```python
from build123d import *

# Parameters (mm, degrees)
SKETCH1_W                  = 25.4
SKETCH1_H                  = 25.4
BOSS_EXTRUDE1_DEPTH        = 6.35
SKETCH2_R                  = 3.175
CUT_EXTRUDE1_DEPTH         = 20.05
F_6_32_TAPPED_HOLE1_REACH  = 31.099
F_6_32_TAPPED_HOLE1_BORE_R = 1.35255


with BuildPart() as part:
    # Sketch1 → Boss-Extrude1 (new body)
    with BuildSketch(Plane(origin=(0, 0, 0), x_dir=(1, 0, 0), z_dir=(0, 1, 0))):
        Rectangle(SKETCH1_W, SKETCH1_H)
    extrude(amount=BOSS_EXTRUDE1_DEPTH)

    # Sketch2 → Cut-Extrude1 (cut, through all)
    with BuildSketch(Plane(origin=(0, 6.35, 0), x_dir=(1, 0, 0), z_dir=(0, 1, 0))):
        with Locations(Location((0, 0, 0), (0, 0, 270))):
            Circle(SKETCH2_R)
    extrude(amount=-CUT_EXTRUDE1_DEPTH, mode=Mode.SUBTRACT)

    # #6-32 Tapped Hole1 bore → #6-32 Tapped Hole1 (cut, up to next)
    with BuildSketch(Plane(origin=(0, 0, -12.7), x_dir=(-1, 0, 0), z_dir=(0, 0, -1)), mode=Mode.PRIVATE) as f_6_32_tapped_hole1_sk1:
        with Locations((0, 3.175)):
            Circle(F_6_32_TAPPED_HOLE1_BORE_R)
    f_6_32_tapped_hole1_tool1 = extrude(f_6_32_tapped_hole1_sk1.sketch, amount=-F_6_32_TAPPED_HOLE1_REACH, mode=Mode.PRIVATE) & part.part
    add(f_6_32_tapped_hole1_tool1.solids().sort_by_distance((0, 3.175, -12.7))[0], mode=Mode.SUBTRACT)


solid = part.part
```
Design review of the part built by this model. Coordinates are the model's own, in mm. Give positions to 0.01 mm unless a question says otherwise; leave off trailing zeros. Loops run counter-clockwise (first coordinate to the right, second up) from the corner with the lowest first, then second, coordinate; pieces in that order, holes last. Notation, with made-up numbers: (-34, 43.5) -> (22, 43.5) arc R18 ccw to (22, 67.5) -> close; hole circle Ø4 at (28, -4). An arc over 180 degrees is marked (long way). One line per item, written item: value.
Q1. We need section C-C on y = 1.5. Give the boundary of the cut face in (x, z) (3 decimals), and give its area (3 significant figures).
Numbers:
outline: (-12.7, -12.7) -> (12.7, -12.7) -> (12.7, 12.7) -> (-12.7, 12.7) -> close; hole circle Ø6.35 at (0, 0)
area: 613 mm^2
Q2. Draft analysis for pull direction Y (two halves, no side actions). For faces 1 (the flat face through (3, 6.35, -3)), 2 (the flat face through (3, 0, -3)), 3 (the flat face through (12.7, 3, 0)), 4 (the cylindrical face through (-0.727, 4.315, -7.855)), state which applies: pulls with the +Y half, pulls with the -Y half, needs draft (parallel to the pull), parting line crosses it, or undercut.
Numbers:
face 1: pulls with the +Y half
face 2: pulls with the -Y half
face 3: needs draft
face 4: undercut
Q3. We need section D-D on z = -3.5. Give the boundary of the cut face in (x, y) (3 decimals), and give its area (3 significant figures).
Numbers:
outline: (-12.7, 0) -> (12.7, 0) -> (12.7, 6.35) -> (-12.7, 6.35) -> close; hole circle Ø2.705 at (0, 3.175)
area: 156 mm^2
Q4. We need section A-A on x = 0. Give the boundary of the cut face in (y, z) (3 decimals), and give its area (3 significant figures).
Numbers:
outline: (0, -12.7) -> (1.822, -12.7) -> (1.822, -3.175) -> (0, -3.175) -> close; (0, 3.175) -> (6.35, 3.175) -> (6.35, 12.7) -> (0, 12.7) -> close; (4.528, -12.7) -> (6.35, -12.7) -> (6.35, -3.175) -> (4.528, -3.175) -> close
area: 95.2 mm^2
Q5. For L1, parallel to Y at x = 0, z = -10; L2, parallel to X at y = 3, z = 0 (3 decimals); L3, parallel to Z at x = -1.25, y = 4.75, list the stretches that pass through material, from the lowest coordinate up.
Numbers:
L1: y = 0 to 1.82, 4.53 to 6.35
L2: x = -12.7 to -3.175, 3.175 to 12.7
L3: z = -12.7 to -2.92, 2.92 to 12.7
Q6. We need section B-B on z = 0. Give the boundary of the cut face in (x, y) (3 decimals).
Numbers:
outline: (-12.7, 0) -> (-3.175, 0) -> (-3.175, 6.35) -> (-12.7, 6.35) -> close; (3.175, 0) -> (12.7, 0) -> (12.7, 6.35) -> (3.175, 6.35) -> close
